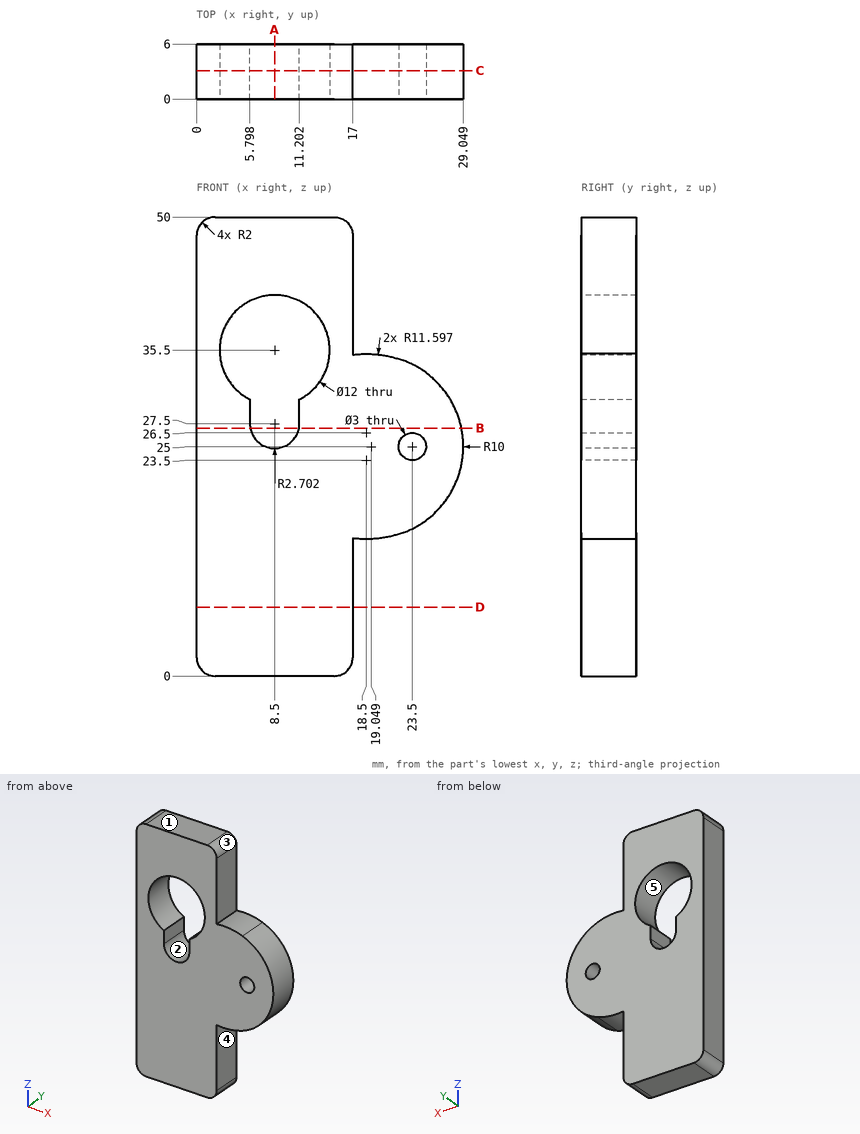
Design review of the part shown in the three views and the two pictorial views. Dimensions are in mm from the part's minimum x, y and z. A direction names the side the tool comes from. Give positions to 0.01 mm unless a question says otherwise; leave off trailing zeros. Write each loop counter-clockwise with the first axis right and the second up, starting at its lowest first coordinate (ties: lowest second). Pieces come first, ordered by that corner, then holes.
Item 1: Insertion check: P1, Ø1, axis at x = 21.5, y = 5, coming from the -Z side (1 decimal); P2, Ø1.5, axis at y = 3.5, z = 13.5, coming from the +X side; P3, Ø1.5, axis at x = 24, y = 4.5, coming from the +Z side (1 decimal). Each pin has a flat end and moves straight along its axis. Give the tip position at first contact, or say it passes through.
Item 2: Take a section at B-B (z = 27). Give the boundary of the cut face in (x, y) (1 decimal), and give its area (3 significant figures).
Item 3: The part is to be moulded in two halves that separate along Z. For the marked faces 3, 4 and 5, say which applies: +Z half, -Z half, draft (parallel to the pull), parting line (faces both ways), or undercut.
Item 4: Take a section at D-D (z = 7.5). Give the boundary of the cut face in (x, y), and give its area (3 significant figures).
Item 5: Take a section at C-C (y = 3.1). Give the number of separate pieces and of enclosed holes in the cut face.
Item 6: Wall thickness on probe 1 along Z at (x, y) = (8.5, 2.5); probe 2 along X at (y, z) = (1.9, 35.5); probe 3 along X at (y, z) = (1.2, 7.5): over which ranges is each line inside the solid? List them lowest first.
Item 7: Machinability: for the marked faces 1 and 2, which of the approach directions +Z, -Z, +X, -X, +Y, -Y give a long, thin tool a straight path to every point of the face, cutting with its end or side? Answer none if there is none.
Item 8: Take a section at A-A (x = 8.5). Give the boundary of the cut face in (y, z), and give its area (3 significant figures).
Established:
1. P1: stops at z = 15.2
1. P2: stops at x = 17
1. P3: stops at z = 34.1
2. outline: (0, 0) - (5.8, 0) - (5.8, 6) - (0, 6) - close; (11.2, 0) - (28.8, 0) - (28.8, 6) - (11.2, 6) - close
2. area: 141 mm2
3. face 3: +Z half
3. face 4: draft
3. face 5: undercut
4. outline: (0, 0) - (17, 0) - (17, 6) - (0, 6) - close
4. area: 102 mm2
5. separate pieces: 1
5. enclosed holes: 2
6. probe 1: z = 0 to 24.8, 41.5 to 50
6. probe 2: x = 0 to 2.5, 14.5 to 17
6. probe 3: x = 0 to 17
7. face 1: +Z, +X, -X, +Y, -Y
7. face 2: +Y, -Y
8. outline: (0, 0) - (6, 0) - (6, 24.8) - (0, 24.8) - close; (0, 41.5) - (6, 41.5) - (6, 50) - (0, 50) - close
8. area: 200 mm2
